Verification items for the finished model (mm, model axes). Give positions to 0.01 mm unless a question says otherwise; leave off trailing zeros. Order: outer loops, then holes, each group sorted by start corner. A loop starts at its lowest first (then second) coordinate and runs counter-clockwise, first axis right, second up. Notation, with made-up numbers: (36, 7) -> (89, 7) arc R20 ccw to (89, 42) -> close; hole circle Ø10 at (53.5, -33). An arc over 180 degrees is marked (long way). Return JSON: item names as keys, results as strings. Group by question number.
(1) Cross-section at B-B on z = -6.25. Enter the section's corners in (x, y), then the cut area to 3 significant figures.
(2) Cross-section at A-A on x = -5. Enter the section's corners in (y, z), then the cut area to 3 significant figures.
(3) Cross-section at C-C on y = 1.7. Enter the section's corners in (x, z), then the cut area to 3 significant figures.
(4) Thickness scan on line 1 along Z through (x, y) = (-5, 1.3); line 2 along X through (y, z) = (0.8, -6.25); line 3 along Z through (x, y) = (-4.25, 1.6). Record the ranges inside material, lowest first.
(5) Release check for a two-part mould opening along X. For faces 1 (the face through (-10, 1, -6)), 2 (the face through (-3.8, 0, -6.2)), 3 (the face through (0, 1, -6)), 4 (the face through (-5.13, 0.99, -5.26)) record: pulls with the +X half, pulls with the -X half, needs draft (parallel to the pull), parting line crosses it, or undercut.
Autodesk Inventor part; units mm, degrees
ref_plane "YZ Plane" through (0, 0, 0) normal (1, 0, 0) x (0, 1, 0)
ref_plane "XZ Plane" through (0, 0, 0) normal (0, 1, 0) x (-1, 0, 0)
ref_plane "XY Plane" through (0, 0, 0) normal (0, 0, 1) x (1, 0, 0)
sketch "Sketch1" plane through (0, 0, 0) normal (0, 1, 0) x (-1, 0, 0)
  line L0 (0, 0) -> (10, 0)
  line L1 (10, 0) -> (10, -12.5)
  line L2 (10, -12.5) -> (0, -12.5)
  line L3 (0, -12.5) -> (0, 0)
  dimension "d0" = 10
  dimension "d1" = 12.5
extrude "Extrusion1" add sketch "Sketch1" along normal blind 2
sketch "Sketch2" plane through (0, 0, 0) normal (0, -1, 0) x (1, 0, 0)
  line L0 (-10, -12.5) -> (-10, 0)
  line L1 (-10, 0) -> (-5, 0)
  line L2 (-5, 0) -> (-5, -6.25)
  line L3 (-5, -6.25) -> (-10, -6.25)
  line L4 (-10, -6.25) -> (-10, 0)
  circle A0 centre (-5, -6.25) radius 1
  point P0 (0, 0)
  dimension "d4" = 5
  dimension "d5" = 6.25
  dimension "d6" = 2
extrude "Extrusion2" cut sketch "Sketch2" against normal blind 2 contours A0 L2 L3 | L3 L2 A0
properties part number "LaserMoutBottom"
Verdict:
{
 "1": {"outline": "(-10, 0) -> (-6, 0) -> (-6, 2) -> (-10, 2) -> close; (-4, 0) -> (0, 0) -> (0, 2) -> (-4, 2) -> close", "area": "16.0 mm²"},
 "2": {"outline": "(0, -12.5) -> (2, -12.5) -> (2, -7.25) -> (0, -7.25) -> close; (0, -5.25) -> (2, -5.25) -> (2, 0) -> (0, 0) -> close", "area": "21.0 mm²"},
 "3": {"outline": "(-10, -12.5) -> (0, -12.5) -> (0, 0) -> (-10, 0) -> close; hole circle Ø2 at (-5, -6.25)", "area": "122 mm²"},
 "4": {"line 1": "-12.5 to -7.25, -5.25 to 0", "line 2": "-10 to -6, -4 to 0", "line 3": "-12.5 to -6.91, -5.59 to 0"},
 "5": {"face 1": "pulls with the -X half", "face 2": "needs draft", "face 3": "pulls with the +X half", "face 4": "undercut"}
}
